Here's how the part is built. I have some questions about the finished solid (model axes, mm). Face numbers are marked on the shaded views. A direction names the side the tool comes from. Coordinates: 2 decimals unless noted, no trailing zeros. Loops run counter-clockwise (first coordinate to the right, second up) from the corner with the lowest first, then second, coordinate; pieces in that order, holes last. Notation, with made-up numbers: (64, 34.5) -> (113, 34.5) arc R33 cw to (113, 64.5) -> close; hole circle Ø2 at (25, 7). An arc over 180 degrees is marked (long way). Answer as a JSON object with one key per item and string values. Group by question number.
Q1. On a 3-axis mill with a long thin cutter (end or side, diameter ignored), from which of +Z, -Z, +X, -X, +Y, -Y can I reach the whole of each face in a straight line? I mean the marked faces 1 and 2. Say none if no direction works.
Q2. I want a section at A-A on x = 2.25. Write out the boundary of the cut face in (y, z), then the cut area to 3 significant figures.
Q3. I want a section at B-B on x = -1.75. Write out the boundary of the cut face in (y, z).
Q4. I need wall thicknesses on line 1 (X direction, y = 11.5, z = 3.75); line 2 (X direction, y = 7.5, z = -10.25); line 3 (Y direction, x = 1, z = -1.25). Which ranges of each line are inside material? Lowest first, please.
Q5. I'm going to push flat-ended pins straight in: pin 1 (2 mm diameter, centred on x = 3, y = 14, fed in from -Z); pin 2 (5.5 mm diameter, centred on y = 18.5, z = -5, fed in from +X); pin 3 (1.4 mm diameter, centred on x = 0.5, y = 11.5, fed in from +Z). Where does each tip first touch, or does it pass through?
Autodesk Inventor part; units mm, degrees
ref_plane "YZ Plane" through (0, 0, 0) normal (1, 0, 0) x (0, 1, 0)
ref_plane "XZ Plane" through (0, 0, 0) normal (0, 1, 0) x (-1, 0, 0)
ref_plane "XY Plane" through (0, 0, 0) normal (0, 0, 1) x (1, 0, 0)
sketch "Sketch1" plane through (0, 0, 0) normal (1, 0, 0) x (0, 1, 0)
  line L0 (0, 0) -> (50, 0)
  line L1 (50, 0) -> (50, -50)
  line L2 (50, -50) -> (0, -50)
  line L3 (0, -50) -> (0, 0)
  circle A0 centre (25, -25) radius 25
  line L4 (25, 0) -> (25, 10)
  line L5 (25, 10) -> (-10, 10)
  line L6 (-10, 10) -> (-10, -25)
  line L7 (-10, -25) -> (0, -25)
  line L8 (25, 0) -> (25, -25)
  line L9 (25, -25) -> (0, -25)
  circle A1 centre (25, -25) radius 20
  circle A2 centre (25, -25) radius 23
  point P0 (50, -25)
  point P1 (25, -50)
  point P2 (2, -25)
  point P3 (25, -2)
  point P4 (5, -25)
  point P5 (25, -5)
  dimension "d0" = 50
  dimension "d1" = 5
  dimension "d2" = 35
  dimension "d3" = 2
extrude "Extrusion1" add sketch "Sketch1" along normal blind 5 contours L3 L7 L6 L5 L4 L0 | L0 A0 L3 | L8 A2 L9 A0 picked at (1.8931, -17.824)
extrude "Extrusion2" add sketch "Sketch1" against normal blind 5 contours L3 L7 L6 L5 L4 L0 | L0 A0 L3 | L8 A2 L9 A0 | L8 A1 L9 A2 picked at (1.8931, -17.824) picked at (4.6117, -17.075)
extrude "Extrusion3" cut sketch "Sketch1" along normal blind 1.8 contours L3 L7 L6 L5 L4 L0
fillet "Fillet1" radius 30 2 edges at (3.4, -10, 10) (-2.5, -10, 10)
sketch "Sketch2" plane through (5, -10, -25) normal (0, 0, -1) x (-1, 0, 0)
  line L0 (20.3331, 29.5099) -> (-16.8181, 29.5099)
  line L1 (-16.8181, 29.5099) -> (-16.8181, -19.9518)
  line L2 (-16.8181, -19.9518) -> (20.3331, -19.9518)
  line L3 (20.3331, -19.9518) -> (20.3331, 29.5099)
  point P0 (5, 10)
extrude "Extrusion4" cut sketch "Sketch2" against normal blind 12
fillet "Fillet4" radius 2 7 edges at (3.4, -9.1719, -13) (-2.5, -9.1719, -13) (5, 22.5, 10) (5, 1.4258, 3.5584) (-5, 22.5, 10) (-5, 1.4258, 3.5584) (5, 13.7528, -4.9376)
properties part number "ESQUINERO_PUERTAS" material "Steel, Mild, Welded"
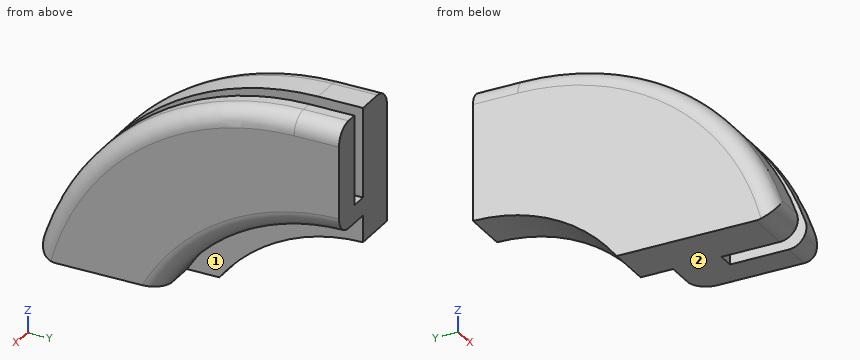
Result set:
{
 "1": {"face 1": "-Z, +X, +Y", "face 2": "-Z, +X, -X, +Y, -Y"},
 "2": {"outline": "(-8.41, -10.36) arc R2 ccw to (-6.51, -13) -> (5.38, -13) arc R23 cw to (25, -2) -> (25, 10) -> (20, 10) arc R30 ccw to start", "area": "460 mm²"},
 "3": {"outline": "(-8.41, -10.36) arc R2 ccw to (-6.51, -13) -> (9, -13) arc R20 cw to (25, -5) -> (25, 10) -> (20, 10) arc R30 ccw to start"},
 "4": {"line 1": "x = -5 to 0, 1.8 to 5", "line 2": "x = -5 to 0", "line 3": "y = 0 to 25"},
 "5": {"pin 1": "stops at z = -5.38", "pin 2": "stops at x = 4.58", "pin 3": "stops at z = 8.91"}
}
